```python
from build123d import *

# Parameters (mm, degrees)
SKETCH_1_W          = 34
SKETCH_1_H          = 49
EXTRUDE_1_DEPTH     = 8
SKETCH_2_W          = 1.5
SKETCH_2_H          = 24
EXTRUDE_2_DEPTH     = 4
SKETCH_3_W          = 1.5
SKETCH_3_H          = 12
SKETCH_3_W_2        = 25
SKETCH_3_H_2        = 13
CUT_EXTRUDE_1_DEPTH = 8
CUT_EXTRUDE_2_REACH = 44.432
SKETCH_4_R          = 2
EXTRUDE_3_DEPTH     = 8
CUT_EXTRUDE_4_DEPTH = 8
SKETCH_6_W          = 4
SKETCH_6_H          = 4
SKETCH_6_W_2        = 3
SKETCH_6_H_2        = 33
EXTRUDE_5_DEPTH     = 12
SKETCH_7_R          = 2.625
EXTRUDE_6_DEPTH     = 3
SKETCH_8_R          = 0.55
CUT_EXTRUDE_5_DEPTH = 4


with BuildPart() as part:
    # 草图1 → 凸台-拉伸1 (new body)
    with BuildSketch(Plane(origin=(0, 0, 0), x_dir=(1, 0, 0), z_dir=(0, 1, 0))):
        Rectangle(SKETCH_1_W, SKETCH_1_H)
    extrude(amount=EXTRUDE_1_DEPTH)

    # 草图2 → 凸台-拉伸2 (add)
    with BuildSketch(Plane(origin=(0, 8, 0), x_dir=(1, 0, 0), z_dir=(0, 1, 0))):
        with Locations((-16.25, 7.5)):
            Rectangle(SKETCH_2_W, SKETCH_2_H)
        with Locations((16.25, 7.5)):
            Rectangle(SKETCH_2_W, SKETCH_2_H)
    extrude(amount=EXTRUDE_2_DEPTH)

    # 草图3 → 切除-拉伸1 (cut)
    with BuildSketch(Plane(origin=(0, 8, 0), x_dir=(1, 0, 0), z_dir=(0, 1, 0))):
        with Locations((-16.25, -18.5)):
            Rectangle(SKETCH_3_W, SKETCH_3_H)
        with Locations((16.25, -18.5)):
            Rectangle(SKETCH_3_W, SKETCH_3_H)
        with Locations((0, -18)):
            Rectangle(SKETCH_3_W_2, SKETCH_3_H_2)
    extrude(amount=-CUT_EXTRUDE_1_DEPTH, mode=Mode.SUBTRACT)

    # 切除-拉伸2: up to this face of the body (flat: up to its plane)
    cut_extrude_2_end = Plane(part.part.faces().sort_by_distance((15.5, 4, 18.5))[0])
    # 草图4 → 切除-拉伸2 (cut, up to the picked face)
    with BuildSketch(Plane.ZY.offset(15.5), mode=Mode.PRIVATE) as cut_extrude_2_sk1:
        with Locations((18.5, 4)):
            Circle(SKETCH_4_R)
    cut_extrude_2_tool1 = split(extrude(cut_extrude_2_sk1.sketch, amount=-CUT_EXTRUDE_2_REACH, mode=Mode.PRIVATE), bisect_by=cut_extrude_2_end, keep=Keep.BOTH, mode=Mode.PRIVATE)
    add(cut_extrude_2_tool1.solids().sort_by(Axis((-15.5, 4, 18.5), (1, 0, 0)))[0], mode=Mode.SUBTRACT)

    # 草图5 → 凸台-拉伸3 (add)
    with BuildSketch(Plane.XZ):
        Polygon((4, 11.5), (-4, 11.5), (-4, 41.5), (-13, 41.5), (-13, 56.5), (13, 56.5), (13, 41.5), (4, 41.5), align=None)
    extrude(amount=-EXTRUDE_3_DEPTH)

    # 草图5<2> → 切除-拉伸4 (cut)
    with BuildSketch(Plane.XZ):
        Polygon((4, 11.5), (-4, 11.5), (-4, 41.5), (-13, 41.5), (-13, 56.5), (13, 56.5), (13, 41.5), (4, 41.5), align=None)
    extrude(amount=-CUT_EXTRUDE_4_DEPTH, mode=Mode.SUBTRACT)

    # 草图6 → 凸台-拉伸5 (add)
    with BuildSketch(Plane.XZ):
        with Locations((-2.25, 8)):
            Rectangle(SKETCH_6_W, SKETCH_6_H)
        with Locations((13.5, -6.5)):
            Rectangle(SKETCH_6_W_2, SKETCH_6_H_2)
        Polygon((-4.25, -19), (-4.25, -19.5), (-4.25, -23), (0, -23), (0, -19.5), (0, -19), align=None)
    extrude(amount=EXTRUDE_5_DEPTH)

    # 草图7 → 凸台-拉伸6 (add)
    with BuildSketch(Plane(origin=(15, 0, 0), x_dir=(0, 0, -1), z_dir=(1, 0, 0))):
        with Locations((12, -7)):
            Circle(SKETCH_7_R)
    extrude(amount=EXTRUDE_6_DEPTH)

    # 草图8 → 切除-拉伸5 (cut)
    with BuildSketch(Plane.ZY.offset(4.25)):
        with Locations((8, -7)):
            Circle(SKETCH_8_R)
        with Locations((-21, -7)):
            Circle(SKETCH_8_R)
    extrude(amount=-CUT_EXTRUDE_5_DEPTH, mode=Mode.SUBTRACT)


solid = part.part
```
Geometry: final body of the model. Coordinates: model frame, mm. A direction names the side the tool comes from. Round coordinates to 2 decimals unless told otherwise and drop trailing zeros. Write each loop counter-clockwise with the first axis right and the second up, starting at its lowest first coordinate (ties: lowest second). Pieces come first, ordered by that corner, then holes. Notation, with made-up numbers: M 37.25,18.25 L 93.25,18.25 A22 ccw 93.25,30.25 Z; hole C 21.5,77 d5. An arc over 180 degrees is marked long. Answer in a Markdown table with one row per item. Add a question column.
(1) Contact query for flat-ended pins moving along their axis: pin 1 (6 mm diameter, centred on x = 12.5, y = -0.5, fed in from +Z); pin 2 (10 mm diameter, centred on x = 6.5, z = 8.5, fed in from +Y); pin 3 (0.9 mm diameter, centred on x = 13.5, y = -4, fed in from -Z); pin 4 (1.2 mm diameter, centred on x = 16, y = 11, fed in from -Z). Output: stop coordinate, or through.
(2) Reachability of faces 4 (the face through (12, -6, -7)), 5 (the face through (-2, -6, 6)), 6 (the face through (16, 10, -19.5)) from +Z, -Z, +X, -X, +Y, -Y: full face, straight path, thin tool, end or side. Return the list, or none.
(3) Draft query along Z for faces 1 (the face through (13, -6, 10)), 2 (the face through (15.5, 2, 17)), 3 (the face through (-2, -6, -19)). Return one class per face: pulls with the +Z half, pulls with the -Z half, needs draft (parallel to the pull), parting line crosses it, or undercut.
(4) Ray query, L1, parallel to X at y = -3, z = -21.5; L2, parallel to X at y = 9.5, z = 0.5; L3, parallel to Y at x = 13.6, z = 18.5. Return the intervals inside material, ascending.
(5) Cut plane A-A, the plane y = -2.75. Return the cut outline in (x, z).
(6) Cut plane C-C, the plane z = 18.5. Return the cut outline in (x, y), then the cut area to 3 significant figures.
(7) Cut plane D-D, the plane x = -13.5. Return the cut outline in (y, z).
(8) Cut plane B-B, the plane z = 8. Return the cut outline in (x, y), then the cut area to 3 significant figures.
Established:
| question | item | result |
|---|---|---|
| 1 | pin 1 | z = 24.5 |
| 1 | pin 2 | y = 8 |
| 1 | pin 3 | z = -23 |
| 1 | pin 4 | z = -19.5 |
| 2 | face 4 | +Z, -Z, -Y |
| 2 | face 5 | -X, -Y |
| 2 | face 6 | -Z, +X, -X, +Y |
| 3 | face 1 | pulls with the +Z half |
| 3 | face 2 | needs draft |
| 3 | face 3 | undercut |
| 4 | L1 | -4.25 to 0, 12 to 15 |
| 4 | L2 | -17 to -15.5, 15.5 to 17 |
| 4 | L3 | 0 to 2, 6 to 8 |
| 5 | outline | M -4.25,-23 L 0,-23 L 0,-19 L -4.25,-19 Z; M -4.25,6 L -0.25,6 L -0.25,10 L -4.25,10 Z; M 12,-23 L 15,-23 L 15,10 L 12,10 Z |
| 6 | outline | M -15.5,0 L -12.5,0 L -12.5,2 L -15.5,2 Z; M -15.5,6 L -12.5,6 L -12.5,8 L -15.5,8 Z; M 12.5,0 L 15.5,0 L 15.5,2 L 12.5,2 Z; M 12.5,6 L 15.5,6 L 15.5,8 L 12.5,8 Z |
| 6 | area | 24.0 mm² |
| 7 | outline | M 0,-24.5 L 8,-24.5 L 8,24.5 L 0,24.5 Z; hole C 4,18.5 d4 |
| 8 | outline | M -17,0 L -4.25,0 L -4.25,-6.45 L -0.25,-6.45 L -0.25,0 L 12,0 L 12,-12 L 15,-12 L 15,0 L 17,0 L 17,8 L -17,8 Z; M -4.25,-12 L -0.25,-12 L -0.25,-7.55 L -4.25,-7.55 Z |
| 8 | area | 352 mm² |
